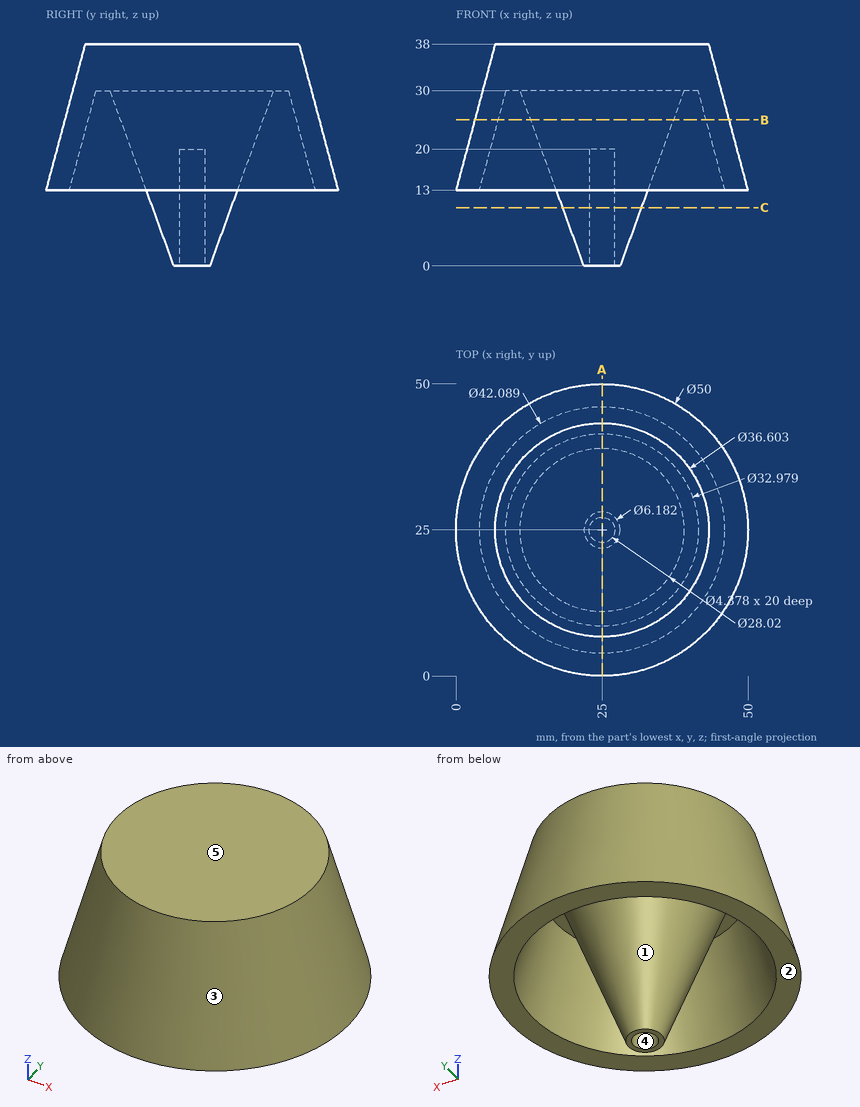
The drawing under review shows one solid part. Ordinate dimensions are in mm from its lowest x, y, z. A direction names the side the tool comes from. Round coordinates to 2 decimals unless told otherwise and drop trailing zeros. Loops run counter-clockwise (first coordinate to the right, second up) from the corner with the lowest first, then second, coordinate; pieces in that order, holes last. Notation, with made-up numbers: (68, 59.25) - (113, 59.25) arc R27 cw to (113, 95.25) - close; hole circle Ø8 at (73, 89.5). An arc over 180 degrees is marked (long way). Use a Markdown table: item, result. Add a question column.
Q1. Insertion check: pin 1 Ø1 at (y, z) = (18.5, 30) entering from -X; pin 2 Ø1 at (y, z) = (35.5, 16.5) entering from +X; pin 3 Ø10 at (x, z) = (25, 10) entering from +Y. Each pin has a flat end and moves straight along its axis. Give the tip position at first contact, or say it passes through.
Q2. The part is to be moulded in two halves that separate along Y. For the marked faces 1, 2 and 3, say which applies: pulls with the +Y half, pulls with the -Y half, needs draft (parallel to the pull), parting line crosses it, or undercut.
Q3. Machinability: for the marked faces 4 and 5, which of the approach directions +Z, -Z, +X, -X, +Y, -Y give a long, thin tool a straight path to every point of the face, cutting with its end or side? Answer none if there is none.
Q4. For probe 1 along X at (y, z) = (25, 14.25) (1 decimal); probe 2 along Y at (x, z) = (17.5, 17) (1 decimal); probe 3 along Z at (x, y) = (38.5, 20.5), list the stretches that pass through material, from the lowest coordinate up.
Q5. Add section B-B (z = 25). State the section outline as (x, y) points (1 decimal).
Q6. Add section A-A (x = 25). State the section outline as (y, z) points (1 decimal), plus the area to 3 significant figures.
Q7. Add section C-C (z = 10). State the section outline as (x, y) points.
Worked answers:
| question | item | result |
|---|---|---|
| 1 | pin 1 | x = 5.4 |
| 1 | pin 2 | x = 46.93 |
| 1 | pin 3 | y = 50 |
| 2 | face 1 | undercut |
| 2 | face 2 | needs draft |
| 2 | face 3 | parting line crosses it |
| 3 | face 4 | -Z |
| 3 | face 5 | +Z, +X, -X, +Y, -Y |
| 4 | probe 1 | 0.3 to 4.3, 16.7 to 22.8, 27.2 to 33.3, 45.7 to 49.7 |
| 4 | probe 2 | 2.3 to 6.5, 19.5 to 30.5, 43.5 to 47.7 |
| 4 | probe 3 | 30 to 38 |
| 5 | outline | circle Ø43.6 at (25, 25); circle Ø24.4 at (25, 25); hole circle Ø35.7 at (25, 25) |
| 6 | outline | (0, 13) - (4, 13) - (8.5, 30) - (11, 30) - (21.9, 0) - (22.8, 0) - (22.8, 20) - (27.2, 20) - (27.2, 0) - (28.1, 0) - (39, 30) - (41.5, 30) - (46, 13) - (50, 13) - (43.3, 38) - (6.7, 38) - close |
| 6 | area | 870 mm² |
| 7 | outline | circle Ø13.46 at (25, 25); hole circle Ø4.38 at (25, 25) |
